Read the model definition and answer for the solid it produces. Units are mm, in the model's axes. Face numbers are marked on the shaded views. Coordinates: 2 decimals unless noted, no trailing zeros. Order: outer loops, then holes, each group sorted by start corner. A loop starts at its lowest first (then second) coordinate and runs counter-clockwise, first axis right, second up. Notation, with made-up numbers: (73.25, -25) -> (80.25, -25) arc R32 cw to (80.25, 1) -> close; hole circle Ø10 at (-6, 73). An arc over 180 degrees is marked (long way). Answer in a Markdown table with one row per item.
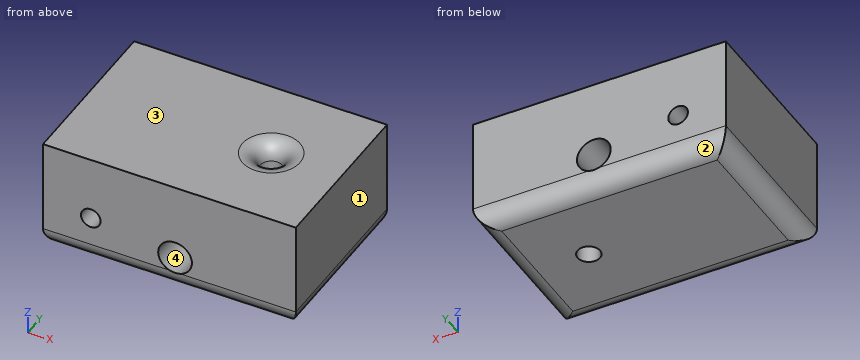
Autodesk Fusion 360 part; units mm, degrees
sketch "Sketch1" plane through (0, 0, 0) normal (0, 0, 1) x (1, 0, 0)
  line L0 (0, 0) -> (114.3, 0)
  line L1 (114.3, 0) -> (114.3, -76.2)
  line L2 (114.3, -76.2) -> (0, -76.2)
  line L3 (0, -76.2) -> (0, 0)
  dimension "d1" = 114.3
  dimension "d2" = 76.2
extrude "Extrude1" add sketch "Sketch1" along normal blind 50.8
sketch "Sketch2" plane through (0, 0, 50.8) normal (0, 0, 1) x (-1, 0, 0)
  line L0 (0, 76.2) -> (-114.3, 76.2)
  line L1 (-114.3, 76.2) -> (-114.3, 0)
  line L2 (-114.3, 0) -> (0, 0)
  line L3 (0, 0) -> (0, 76.2)
  circle A0 centre (-82.55, 38.1) radius 5.08
  dimension "d5" = 10.16
  dimension "d6" = 38.1
  dimension "d7" = 31.75
extrude "Extrude2" cut sketch "Sketch2" against normal blind 50.8 contours A0
fillet "Fillet1" radius 7.9756 1 edges at (87.2862, -39.937, 50.8)
fillet "Fillet2" radius 8.4339 4 edges at (114.3, -38.1, 0) (57.15, -76.2, 0) (0, -38.1, 0) (57.15, 0, 0)
sketch "Sketch3" plane through (0, -76.2, 0) normal (0, -1, 0) x (1, 0, 0)
  line L0 (0, 8.4339) -> (114.3, 8.4339)
  line L1 (114.3, 8.4339) -> (114.3, 50.8)
  line L2 (114.3, 50.8) -> (0, 50.8)
  line L3 (0, 50.8) -> (0, 8.4339)
  circle A0 centre (21.59, 21.59) radius 4.445
  line L4 (8.4339, 0) -> (105.8661, 0)
  circle A1 centre (59.69, 15.6948) radius 7.62
  dimension "d20" = 8.89
  dimension "d21" = 21.59
  dimension "d22" = 21.59
  dimension "d23" = 15.24
  dimension "d24" = 59.69
extrude "Extrude4" cut sketch "Sketch3" against normal blind 76.2 contours L0 A1 | L0 A1
extrude "Extrude5" cut sketch "Sketch3" against normal blind 76.2 contours A0
Q1. The part is cut by section C-C (y = -11). Write down the section's boundary in (x, z) (3 decimals), then the cut area to 3 significant figures.
Outcome:
| item | result |
|---|---|
| outline | (0, 8.434) arc R8.434 ccw to (8.434, 0) -> (105.866, 0) arc R8.434 ccw to (114.3, 8.434) -> (114.3, 50.8) -> (0, 50.8) -> close; hole circle Ø8.89 at (21.59, 21.59); hole circle Ø15.24 at (59.69, 15.695) |
| area | 5,530 mm² |
Q2. The part is cut by section D-D (x = 82.55). Write down the section's boundary in (y, z).
Outcome:
| item | result |
|---|---|
| outline | (-76.2, 8.43) arc R8.43 ccw to (-67.77, 0) -> (-43.18, 0) -> (-43.18, 42.82) arc R7.98 ccw to (-51.16, 50.8) -> (-76.2, 50.8) -> close; (-33.02, 0) -> (-8.43, 0) arc R8.43 ccw to (0, 8.43) -> (0, 50.8) -> (-25.04, 50.8) arc R7.98 ccw to (-33.02, 42.82) -> close |
Q3. Consider line 1 (X direction, y = -7, z = 15.5); line 2 (Z direction, x = 59.69, y = -28); line 3 (X direction, y = -36, z = 21). Determine where each line is inside the solid, lowest interval first.
Outcome:
| item | result |
|---|---|
| line 1 | 0 to 52.07, 67.31 to 114.3 |
| line 2 | 0 to 8.07, 23.31 to 50.8 |
| line 3 | 0 to 17.18, 26 to 54.22, 65.16 to 77.92, 87.18 to 114.3 |
Q4. For a pull along Z with two mould halves and no side action, classify the marked faces 1, 2, 3 and 4 as pulls with the +Z half, pulls with the -Z half, needs draft (parallel to the pull), parting line crosses it, or undercut.
Outcome:
| item | result |
|---|---|
| face 1 | needs draft |
| face 2 | pulls with the -Z half |
| face 3 | pulls with the +Z half |
| face 4 | undercut |
Q5. The part is cut by section A-A (x = 21.59). Write down the section's boundary in (y, z) (3 decimals), then the cut area to 3 significant figures.
Outcome:
| item | result |
|---|---|
| outline | (-76.2, 8.434) arc R8.434 ccw to (-67.766, 0) -> (-8.434, 0) arc R8.434 ccw to (0, 8.434) -> (0, 17.145) -> (-76.2, 17.145) -> close; (-76.2, 26.035) -> (0, 26.035) -> (0, 50.8) -> (-76.2, 50.8) -> close |
| area | 3,160 mm² |
Q6. The part is cut by section B-B (z = 21.59). Write down the section's boundary in (x, y) (3 decimals).
Outcome:
| item | result |
|---|---|
| outline | (0, -76.2) -> (17.145, -76.2) -> (17.145, 0) -> (0, 0) -> close; (26.035, -76.2) -> (54.862, -76.2) -> (54.862, 0) -> (26.035, 0) -> close; (64.518, -76.2) -> (114.3, -76.2) -> (114.3, 0) -> (64.518, 0) -> close; hole circle Ø10.16 at (82.55, -38.1) |
